Verification items for the finished model (mm, model axes). A direction names the side the tool comes from. Give positions to 0.01 mm unless a question says otherwise; leave off trailing zeros. Order: outer loops, then holes, each group sorted by start corner. A loop starts at its lowest first (then second) coordinate and runs counter-clockwise, first axis right, second up. Notation, with made-up numbers: (59.5, 12.25) - (117.5, 12.25) arc R12 ccw to (117.5, 30.25) - close; hole circle Ø3 at (-4, 39.25). An arc over 180 degrees is marked (long way). Answer as a JSON object with one key per item and string values. Group by question number.
(1) Mould release check, pull along X, two halves, no side actions. Record for faces 3 (the face through (-43, 7.62, -3)), 4 (the face through (28.995, 3.757, 37.814)), 5 (the face through (-37.42, 5.81, 21.55)): +X half, -X half, draft (parallel to the pull), parting line (faces both ways), or undercut.
(2) Section check B-B (x = 5). Record the boundary of the cut face in (y, z).
(3) Depth check by flat-ended pin: pin 1 Ø0.8 at (y, z) = (6, 44.5) entering from +X; pin 2 Ø1.3 at (y, z) = (6, -44) entering from +X; pin 3 Ø2 at (y, z) = (5, -44) entering from -X. Enter the tip coordinate at first touch or a pass-through.
(4) Access from +Z, -Z, +X, -X, +Y, -Y to the whole of each face (thin tool, end or side, straight path). Record for faces 1 (the face through (37.27, 2.4, 24.39)), 2 (the face through (41.2, 3.88, -22.03)).
(5) Section check A-A (z = 0). Record the boundary of the cut face in (x, y).
(6) Thickness scan on line 1 (Z direction, x = -1.5, y = 5.75); line 2 (Y direction, x = 0, z = 42.85); line 3 (X direction, y = 5.75, z = -22). Record the ranges inside material, lowest first.
```python
from build123d import *

# Parameters (mm, degrees)
SKETCH2_R           = 47.6504
SKETCH2_R_2         = 41.91
BOSS_EXTRUDE1_DEPTH = 7.62
CUT_EXTRUDE1_DEPTH  = 1.27
SKETCH6_R           = 1.524
CUT_EXTRUDE2_DEPTH  = 6.223
CIRPATTERN1_COUNT   = 6


with BuildPart() as part:
    # Sketch2 → Boss-Extrude1 (new body)
    with BuildSketch(Plane(origin=(0, 0, 0), x_dir=(1, 0, 0), z_dir=(0, 1, 0))):
        with Locations(Location((0, 0, 0), (0, 0, 90))):
            Circle(SKETCH2_R)
        with Locations(Location((0, 0, 0), (0, 0, 90))):
            Circle(SKETCH2_R_2, mode=Mode.SUBTRACT)
    extrude(amount=BOSS_EXTRUDE1_DEPTH)

    # Sketch4 → Cut-Extrude1 (cut, symmetric)
    with BuildSketch(Plane.XY.offset(44.45)):
        Polygon((-1.651, 0.950384117), (0, 0.950384117), (0, 6.669615883), (-1.651, 6.669615883), (-3.302, 3.81), align=None)
        Polygon((0, 6.669615883), (0, 0.950384117), (1.651, 0.950384117), (3.302, 3.81), (1.651, 6.669615883), align=None)
        Polygon((0, 7.62), (0, 6.669615883), (1.651, 6.669615883), (3.302, 3.81), (3.302, 7.62), align=None)
        Polygon((-1.651, 6.669615883), (0, 6.669615883), (0, 7.62), (-3.302, 7.62), (-3.302, 3.81), align=None)
    cut_extrude1 = extrude(amount=CUT_EXTRUDE1_DEPTH, both=True, mode=Mode.SUBTRACT)

    # Sketch6 → Cut-Extrude2 (cut, symmetric)
    with BuildSketch(Plane.XY.offset(44.45)):
        with Locations((0, 3.81)):
            Circle(SKETCH6_R)
    cut_extrude2 = extrude(amount=CUT_EXTRUDE2_DEPTH, both=True, mode=Mode.SUBTRACT)

    # CirPattern1: Cut-Extrude1, Cut-Extrude2 ×6 about axis
    cirpattern1_axis = Axis((0, 0, 0), (0, 1, 0))
    add([cut_extrude1.rotate(cirpattern1_axis, i * 360 / CIRPATTERN1_COUNT) for i in range(1, CIRPATTERN1_COUNT)], mode=Mode.SUBTRACT)
    add([cut_extrude2.rotate(cirpattern1_axis, i * 360 / CIRPATTERN1_COUNT) for i in range(1, CIRPATTERN1_COUNT)], mode=Mode.SUBTRACT)


solid = part.part
```
Solutions:
{
 "1": {"face 3": "draft", "face 4": "parting line", "face 5": "undercut"},
 "2": {"outline": "(0, -47.39) - (7.62, -47.39) - (7.62, -41.61) - (0, -41.61) - close; (0, 41.61) - (7.62, 41.61) - (7.62, 47.39) - (0, 47.39) - close"},
 "3": {"pin 1": "stops at x = 18.05", "pin 2": "stops at x = 19.78", "pin 3": "stops at x = -20.53"},
 "4": {"face 1": "+Y", "face 2": "none"},
 "5": {"outline": "(-47.65, 0) - (-41.91, 0) - (-41.91, 7.62) - (-47.65, 7.62) - close; (41.91, 0) - (47.65, 0) - (47.65, 7.62) - (41.91, 7.62) - close"},
 "6": {"line 1": "z = -47.63 to -45.72, -43.18 to -41.88, 41.88 to 43.18, 45.72 to 47.63", "line 2": "y = 0 to 2.29, 5.33 to 7.62", "line 3": "x = -42.27 to -40.09, -37.16 to -35.67, 35.67 to 37.16, 40.09 to 42.27"}
}
